Autodesk Inventor part; units mm, degrees
ref_plane "YZ Plane" through (0, 0, 0) normal (1, 0, 0) x (0, 1, 0)
ref_plane "XZ Plane" through (0, 0, 0) normal (0, 1, 0) x (-1, 0, 0)
ref_plane "XY Plane" through (0, 0, 0) normal (0, 0, 1) x (1, 0, 0)
sketch "Sketch1" plane through (0, 0, 0) normal (1, 0, 0) x (0, 1, 0)
  line L0 (0, 0) -> (6.35, 0)
  line L1 (6.35, 0) -> (6.35, 12.7)
  line L2 (0, 0) -> (0, 12.7)
  line L3 (0, 12.7) -> (-3.175, 12.7)
  line L4 (-3.175, 12.7) -> (-3.175, -34.29)
  line L5 (6.35, 12.7) -> (9.525, 12.7)
  line L6 (9.525, 12.7) -> (9.525, -34.29)
  line L7 (9.525, -34.29) -> (-3.175, -34.29)
  dimension "d0" = 6.35
  dimension "d1" = 12.7
  dimension "d2" = 3.175
  dimension "d3" = 46.99
  dimension "d4" = 3.175
extrude "Extrusion1" add sketch "Sketch1" along normal blind 12.7
sketch "Sketch2" plane through (0, 9.525, 12.7) normal (0, 1, 0) x (1, 0, 0)
  line L0 (12.7, 0) -> (12.7, 46.99)
  line L1 (0, 12.7) -> (12.7, 0)
  circle A0 centre (6.35, 6.35) radius 2.1082
  dimension "d7" = 4.2164
extrude "Extrusion2" cut sketch "Sketch2" against normal blind 41.275
sketch "Sketch3" plane through (0, 9.525, 12.7) normal (0, 1, 0) x (1, 0, 0)
  line L0 (12.7, 0) -> (12.7, 46.99)
  line L1 (12.7, 46.99) -> (12.7, 34.29)
  line L2 (0, 0) -> (0, 46.99)
  line L3 (12.7, 34.29) -> (0, 46.99)
  circle A0 centre (6.35, 40.64) radius 2.1082
  point P0 (0, 12.7)
  dimension "d10" = 12.7
  dimension "d11" = 4.2164
extrude "Extrusion3" cut sketch "Sketch3" against normal blind 33.3375
fillet "Fillet5" radius 6.35 2 edges at (0, 3.175, -34.29) (12.7, 3.175, -34.29)
sketch "Sketch6" plane through (0, 0, 0) normal (0, 0, 1) x (1, 0, 0)
  line L0 (0, 0) -> (12.7, 0)
  line L1 (0, 6.35) -> (12.7, 6.35)
  line L2 (0, 0) -> (12.7, 0)
  line L3 (12.7, 0) -> (12.7, 6.35)
  line L4 (12.7, 6.35) -> (0, 6.35)
  line L5 (0, 6.35) -> (0, 0)
extrude "Extrusion6" cut sketch "Sketch6" against normal blind 6.35
fillet "Fillet6" radius 6.35 6 edges at (0, 7.9375, 12.7) (0, -1.5875, 12.7) (0, 3.175, -6.35) (12.7, 7.9375, 12.7) (12.7, -1.5875, 12.7) (12.7, 3.175, -6.35)
properties part number "wing bar v2"
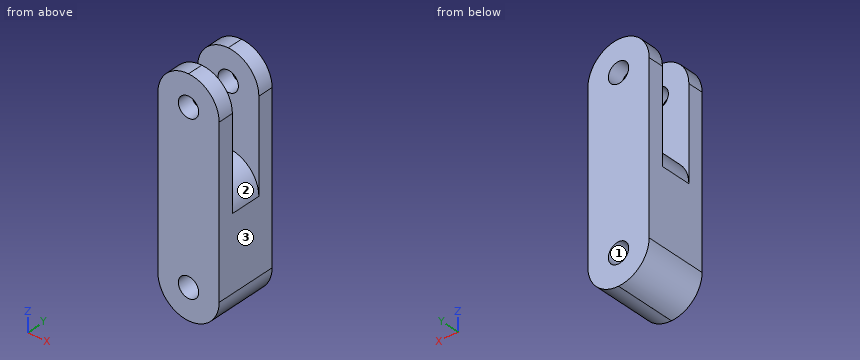
Can you work these out from the model? Positions are in its coordinate system, mm. Face numbers are marked on the shaded views. Give positions to 0.01 mm unless a question says otherwise; leave off trailing zeros. Loops run counter-clockwise (first coordinate to the right, second up) from the corner with the lowest first, then second, coordinate; pieces in that order, holes last. Notation, with made-up numbers: M -32,7.25 L 18,7.25 A19 cw 18,19.25 Z; hole C -2,-2 d6. An arc over 180 degrees is marked long. Answer in a Markdown table with one row per item.
1. For pin 1 Ø3 at (x, y) = (10, 3.5) entering from +Z, with a flat end and sliding along its axis, tell me the tip position at first contact or that it passes through.
Taken from the geometry:
| item | result |
|---|---|
| pin 1 | stops at z = -6.72 |
2. Suppose I cut it at A-A on x = 5.75. Write out the boundary of the cut face in (y, z) (3 decimals).
Taken from the geometry:
| item | result |
|---|---|
| outline | M -3.175,-34.262 L 9.525,-34.262 L 9.525,-29.961 L -3.175,-29.961 Z; M -3.175,-25.919 L 9.525,-25.919 L 9.525,4.329 L 6.35,4.329 L 6.35,-6.378 L 0,-6.378 L 0,4.329 L -3.175,4.329 Z; M -3.175,8.371 L 0,8.371 L 0,12.672 L -3.175,12.672 Z; M 6.35,8.371 L 9.525,8.371 L 9.525,12.672 L 6.35,12.672 Z |
3. Thinking about a two-plate mould opening in Z: for the marked faces 1, 2 and 3, which applies, released by +Z, released by -Z, zero draft, split by the parting line, or undercut?
Taken from the geometry:
| item | result |
|---|---|
| face 1 | undercut |
| face 2 | released by +Z |
| face 3 | zero draft |
4. Suppose I cut it at C-C on x = 2.5. Write out the boundary of the cut face in (y, z) (3 decimals).
Taken from the geometry:
| item | result |
|---|---|
| outline | M -3.175,-32.99 L 9.525,-32.99 L 9.525,11.4 L 6.35,11.4 L 6.35,-7.65 L 0,-7.65 L 0,11.4 L -3.175,11.4 Z |
5. Suppose I cut it at D-D on y = 7. Count the separate pieces of the cut face and the enclosed holes in it, plus the area to 3 significant figures.
Taken from the geometry:
| item | result |
|---|---|
| separate pieces | 1 |
| enclosed holes | 2 |
| area | 534 mm² |
6. If I drill on line 1 along Z through (x, y) = (6.35, -2.1); line 2 along Y through (x, z) = (6.5, -3.5) (3 decimals); line 3 along X through (y, z) = (5.75, -27.94), over which ranges is the centre line in solid material (lowest first)?
Taken from the geometry:
| item | result |
|---|---|
| line 1 | z = -34.29 to -30.05, -25.83 to 4.24, 8.46 to 12.7 |
| line 2 | y = -3.175 to 0, 6.35 to 9.525 |
| line 3 | x = 0 to 4.24, 8.46 to 12.7 |
